from build123d import *

# Parameters (mm, degrees)
PLAT_W                      = 60
PLAT_H                      = 15
EL_MENT_M_CANO_SOUD_1_DEPTH = 120
ESQUISSE2_R                 = 10
ENL_V_MAT_EXTRU_1_DEPTH     = 20


with BuildPart() as part:
    # plat → Elément mécano-soudé1 (new body)
    with BuildSketch(Plane.YZ.offset(-60)):
        Rectangle(PLAT_W, PLAT_H)
    extrude(amount=EL_MENT_M_CANO_SOUD_1_DEPTH)

    # Esquisse2 → Enlèv. mat.-Extru.1 (cut)
    with BuildSketch(Plane.XY.offset(7.5)):
        with Locations((-20, 0)):
            Circle(ESQUISSE2_R)
    extrude(amount=-ENL_V_MAT_EXTRU_1_DEPTH, mode=Mode.SUBTRACT)


solid = part.part
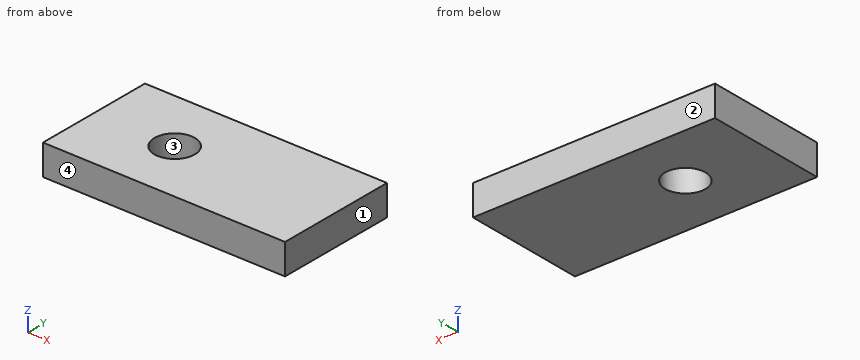
Here's how the part is built. I have some questions about the finished solid (model axes, mm). Face numbers are marked on the shaded views. Give positions to 0.01 mm unless a question says otherwise; leave off trailing zeros. Order: outer loops, then holes, each group sorted by start corner. A loop starts at its lowest first (then second) coordinate and runs counter-clockwise, first axis right, second up. Notation, with made-up numbers: M 37,80 L 83,80 A8 ccw 83,87 Z; hole C 58,63.5 d8. An arc over 180 degrees is marked long. Answer as a JSON object with one key per item and string values. Group by question number.
1) Suppose I cut it at A-A, the plane y = 0. Write out the boundary of the cut face in (x, z).
2) Suppose I cut it at B-B, the plane z = 4.5. Write out the boundary of the cut face in (x, y).
3) Please list where these lines run through material, in increasing order: L1, parallel to Y at x = -20, z = 0; L2, parallel to X at y = 3.5, z = 2.5; L3, parallel to Y at x = -25.5, z = -4.25. Write a range as [from, to].
4) We'd pull the mould along Y, two halves only. Please class the marked faces 1, 2, 3 and 4: pulls with the +Y half, pulls with the -Y half, needs draft (parallel to the pull), parting line crosses it, or undercut.
5) I'm going to push a flat-ended pin straight in: pin 1 Ø12 at (x, y) = (-20, 0) entering from +Z. Where does the tip first touch, or does it pass through?
6) Suppose I cut it at C-C, the plane x = -20. Write out the boundary of the cut face in (y, z).
Results found:
{
 "1": {"outline": "M -60,-7.5 L -30,-7.5 L -30,7.5 L -60,7.5 Z; M -10,-7.5 L 60,-7.5 L 60,7.5 L -10,7.5 Z"},
 "2": {"outline": "M -60,-30 L 60,-30 L 60,30 L -60,30 Z; hole C -20,0 d20"},
 "3": {"L1": "[-30, -10], [10, 30]", "L2": "[-60, -29.37], [-10.63, 60]", "L3": "[-30, -8.35], [8.35, 30]"},
 "4": {"face 1": "needs draft", "face 2": "pulls with the +Y half", "face 3": "undercut", "face 4": "pulls with the -Y half"},
 "5": {"pin 1": "through"},
 "6": {"outline": "M -30,-7.5 L -10,-7.5 L -10,7.5 L -30,7.5 Z; M 10,-7.5 L 30,-7.5 L 30,7.5 L 10,7.5 Z"}
}
